The model under review builds one solid part; all positions refer to its coordinate system, in mm. A direction names the side the tool comes from. Give positions to 0.01 mm unless a question says otherwise; leave off trailing zeros. Order: outer loops, then holes, each group sorted by start corner. A loop starts at its lowest first (then second) coordinate and runs counter-clockwise, first axis right, second up.
Autodesk Inventor part; units mm, degrees
ref_plane "YZ Plane" through (0, 0, 0) normal (1, 0, 0) x (0, 1, 0)
ref_plane "XZ Plane" through (0, 0, 0) normal (0, 1, 0) x (-1, 0, 0)
ref_plane "XY Plane" through (0, 0, 0) normal (0, 0, 1) x (1, 0, 0)
sketch "Sketch1" plane through (0, 0, 0) normal (0, 1, 0) x (-1, 0, 0)
  line L0 (-50, 60) -> (50, 60)
  line L1 (50, 60) -> (50, -60)
  line L2 (50, -60) -> (-50, -60)
  line L3 (-50, -60) -> (-50, 60)
  line L4 (-50, 60) -> (50, -60) construction
  line L5 (50, 60) -> (-50, -60) construction
  line L6 (30, 40) -> (-30, 40)
  line L7 (-30, 40) -> (-30, -40)
  line L8 (-30, -40) -> (30, -40)
  line L9 (30, -40) -> (30, 40)
  line L10 (30, 40) -> (-30, -40) construction
  line L11 (-30, 40) -> (30, -40) construction
  point P0 (0, 0)
  dimension "d0" = 100
  dimension "d1" = 120
  dimension "d2" = 60
  dimension "d3" = 80
extrude "Extrusion1" add sketch "Sketch1" along normal blind 20
sketch "Sketch2" plane through (0, 20, 0) normal (0, 1, 0) x (1, 0, 0)
  circle A0 centre (-40, 50) radius 4.5
  line L0 (-50, 60) -> (-50, -60)
  circle A1 centre (-40, 0) radius 4.5
  circle A2 centre (-40, -50) radius 4.5
  line L1 (0, -4.5) -> (0, 7.1494) construction
  circle A3 centre (40, 50) radius 4.5
  circle A4 centre (40, 0) radius 4.5
  circle A5 centre (40, -50) radius 4.5
  point P0 (0, 0)
  dimension "d6" = 9
  dimension "d7" = 10
  dimension "d8" = 50
  dimension "d9" = 9
  dimension "d10" = 9
  dimension "d11" = 50
extrude "Extrusion2" cut sketch "Sketch2" against normal through all
sketch "Sketch3" plane through (0, 20, 0) normal (0, 1, 0) x (1, 0, 0)
  circle A0 centre (-40, 50) radius 4.5
  circle A1 centre (-40, 50) radius 7.5
  circle A2 centre (-40, 0) radius 4.5
  circle A3 centre (-40, 0) radius 7.5
  circle A4 centre (-40, -50) radius 4.5
  circle A5 centre (-40, -50) radius 7.5
  circle A6 centre (40, -50) radius 4.5
  circle A7 centre (40, -50) radius 7.5
  circle A8 centre (40, 0) radius 4.5
  circle A9 centre (40, 0) radius 7.5
  circle A10 centre (40, 50) radius 4.5
  circle A11 centre (40, 50) radius 7.5
  point P0 (0, 0)
  dimension "d14" = 15
  dimension "d15" = 15
  dimension "d16" = 15
  dimension "d17" = 15
  dimension "d18" = 15
  dimension "d19" = 15
extrude "Extrusion3" cut sketch "Sketch3" against normal blind 9
fillet "Fillet1" radius 10 4 edges at (-30, 10, -40) (-30, 10, 40) (30, 10, 40) (30, 10, -40)
chamfer "Chamfer1" distance 4 angle 45 4 edges at (50, 10, 60) (-50, 10, 60) (-50, 10, -60) (50, 10, -60)
properties part number "peca3"
1. Take a section at A-A (x = 14). Write out the cut boundary in (y, z), and give its area (3 significant figures).
2. Draft analysis for pull direction X (two halves, no side actions). For faces 1 (the flat face through (48, 10, -58)), 2 (the cylindrical face through (-32.846, 15.563, -2.253)), 3 (the flat face through (-33, 20, 14)), state which applies: pulls with the +X half, pulls with the -X half, needs draft (parallel to the pull), parting line crosses it, or undercut.
3. To check wall thickness, follow line 1 (X direction, y = 8.75, z = -50); line 2 (X direction, y = 17.5, z = 50); line 3 (X direction, y = 7.25, z = 0). State the ranges of each line that lie inside material, in increasing order.
4. Insertion check: pin 1 (13.5 mm diameter, centred on x = -40, z = 50, fed in from +Y); pin 2 (7 mm diameter, centred on x = 40, z = 0, fed in from +Y). Each pin has a flat end and moves straight along its axis. Give the tip position at first contact, or say it passes through.
5. Take a section at C-C (y = 12.75). Write out the cut boundary in (x, z), and give its area (3 significant figures).
6. Take a section at D-D (x = 40). Write out the cut boundary in (y, z), and give its area (3 significant figures).
7. Take a section at B-B (z = 38). Write out the cut boundary in (x, y), and give its area (3 significant figures).
8. For faces 4 (the flat face through (0, 10, -40)), 5 (the flat face through (48, 10, 58)), 6 (the cylindrical face through (-41.63, 15.56, 57.32)), list the 3-axis set-ups (+Z, -Z, +X, -X, +Y, -Y) from which the entire face can be reached by the end or side of a thin tool; tool diameter is ignored.
Answer:
1. outline: (0, -60) - (20, -60) - (20, -40) - (0, -40) - close; (0, 40) - (20, 40) - (20, 60) - (0, 60) - close
1. area: 800 mm2
2. face 1: pulls with the +X half
2. face 2: undercut
2. face 3: needs draft
3. line 1: x = -50 to -44.5, -35.5 to 35.5, 44.5 to 50
3. line 2: x = -50 to -47.5, -32.5 to 32.5, 47.5 to 50
3. line 3: x = -50 to -44.5, -35.5 to -30, 30 to 35.5, 44.5 to 50
4. pin 1: stops at y = 11
4. pin 2: passes through
5. outline: (-50, -56) - (-46, -60) - (46, -60) - (50, -56) - (50, 56) - (46, 60) - (-46, 60) - (-50, 56) - close; hole circle Ø15 at (-40, -50); hole circle Ø15 at (-40, 0); hole circle Ø15 at (-40, 50); hole (-30, -30) arc R10 ccw to (-20, -40) - (20, -40) arc R10 ccw to (30, -30) - (30, 30) arc R10 ccw to (20, 40) - (-20, 40) arc R10 ccw to (-30, 30) - close; hole circle Ø15 at (40, -50); hole circle Ø15 at (40, 0); hole circle Ø15 at (40, 50)
5. area: 6,190 mm2
6. outline: (0, -60) - (20, -60) - (20, -57.5) - (11, -57.5) - (11, -54.5) - (0, -54.5) - close; (0, -45.5) - (11, -45.5) - (11, -42.5) - (20, -42.5) - (20, -7.5) - (11, -7.5) - (11, -4.5) - (0, -4.5) - close; (0, 4.5) - (11, 4.5) - (11, 7.5) - (20, 7.5) - (20, 42.5) - (11, 42.5) - (11, 45.5) - (0, 45.5) - close; (0, 54.5) - (11, 54.5) - (11, 57.5) - (20, 57.5) - (20, 60) - (0, 60) - close
6. area: 1,700 mm2
7. outline: (-50, 0) - (-26, 0) - (-26, 20) - (-50, 20) - close; (26, 0) - (50, 0) - (50, 20) - (26, 20) - close
7. area: 960 mm2
8. face 4: +Y, -Y
8. face 5: +Z, +X, +Y, -Y
8. face 6: +Y
